Geometry check sheet. Reference: the model listing, model coordinates, mm. A direction names the side the tool comes from. Round coordinates to 2 decimals unless told otherwise and drop trailing zeros. Write each loop counter-clockwise with the first axis right and the second up, starting at its lowest first coordinate (ties: lowest second). Pieces come first, ordered by that corner, then holes. Notation, with made-up numbers: (81.25, 51) -> (132.25, 51) arc R32 ccw to (132.25, 81) -> close; hole circle Ø1 at (23.25, -12). An arc over 180 degrees is marked (long way). Use a Markdown table: item, result.
```python
from build123d import *

# Parameters (mm, degrees)
CROQUIS1_W              = 29
CROQUIS1_H              = 46
SALIENTE_EXTRUIR1_DEPTH = 4
CROQUIS2_W              = 5
CROQUIS2_H              = 29
SALIENTE_EXTRUIR2_DEPTH = 7
CROQUIS3_W              = 5
CROQUIS3_H              = 29
SALIENTE_EXTRUIR3_DEPTH = 21
CROQUIS4_W              = 29
CROQUIS4_H              = 15
SALIENTE_EXTRUIR4_DEPTH = 28
CROQUIS5_R              = 1.5
CORTAR_EXTRUIR1_DEPTH   = 28
CROQUIS6_W              = 28
CROQUIS6_H              = 10
CORTAR_EXTRUIR2_DEPTH   = 60
CORTAR_EXTRUIR3_START   = -5
CROQUIS7_W              = 4.510634874
CROQUIS7_H              = 12.04330307
CORTAR_EXTRUIR3_DEPTH   = 60
CORTAR_EXTRUIR4_START   = -5
CROQUIS8_W              = 3.464680309
CROQUIS8_H              = 12
CORTAR_EXTRUIR4_DEPTH   = 60


with BuildPart() as part:
    # Croquis1 → Saliente-Extruir1 (new body)
    with BuildSketch(Plane(origin=(0, 0, 0), x_dir=(0, 1, 0), z_dir=(0, 0, 1))):
        Rectangle(CROQUIS1_W, CROQUIS1_H)
    extrude(amount=SALIENTE_EXTRUIR1_DEPTH)



with BuildPart() as body_2:
    # Croquis2 → Saliente-Extruir2 (new body)
    with BuildSketch(Plane.XY.offset(4)):
        with Locations((-25.5, 0)):
            Rectangle(CROQUIS2_W, CROQUIS2_H)
    extrude(amount=SALIENTE_EXTRUIR2_DEPTH)


with BuildPart() as part_1:
    add(part.part)

    add(body_2.part)  # Saliente-Extruir3 merges body 2
    # Croquis3 → Saliente-Extruir3 (add)
    with BuildSketch(Plane(origin=(0, 0, 4), x_dir=(1, 0, 0), z_dir=(0, 0, -1))):
        with Locations((-25.5, 0)):
            Rectangle(CROQUIS3_W, CROQUIS3_H)
    extrude(amount=SALIENTE_EXTRUIR3_DEPTH)

    # Croquis4 → Saliente-Extruir4 (add)
    with BuildSketch(Plane(origin=(-28, 0, 0), x_dir=(0, -1, 0), z_dir=(-1, 0, 0))):
        with Locations((0, -9.5)):
            Rectangle(CROQUIS4_W, CROQUIS4_H)
    extrude(amount=-SALIENTE_EXTRUIR4_DEPTH)

    # Croquis5 → Cortar-Extruir1 (cut)
    with BuildSketch(Plane.XY.offset(4)):
        with Locations((17.5, -9)):
            Circle(CROQUIS5_R)
        with Locations((17.5, 9)):
            Circle(CROQUIS5_R)
        Polygon((-18.5, 0), (-18.5, -6), (4.3, -6), (4.3, 6), (-18.5, 6), align=None)
    extrude(amount=-CORTAR_EXTRUIR1_DEPTH, mode=Mode.SUBTRACT)

    # Croquis6 → Cortar-Extruir2 (cut)
    with BuildSketch(Plane(origin=(0, 14.5, 0), x_dir=(1, 0, 0), z_dir=(0, 1, 0))):
        with Locations((-14, 12)):
            Rectangle(CROQUIS6_W, CROQUIS6_H)
    extrude(amount=-CORTAR_EXTRUIR2_DEPTH, mode=Mode.SUBTRACT)

    # Croquis7 → Cortar-Extruir3 (cut)
    with BuildSketch(Plane.XY.offset(4).offset(CORTAR_EXTRUIR3_START)):
        with Locations((-20.769799618, -0.048913864)):
            Rectangle(CROQUIS7_W, CROQUIS7_H)
    extrude(amount=-CORTAR_EXTRUIR3_DEPTH, mode=Mode.SUBTRACT)

    # Croquis8 → Cortar-Extruir4 (cut)
    with BuildSketch(Plane.XY.offset(4).offset(CORTAR_EXTRUIR4_START)):
        with Locations((-18.492763456, 0)):
            Rectangle(CROQUIS8_W, CROQUIS8_H)
    extrude(amount=-CORTAR_EXTRUIR4_DEPTH, mode=Mode.SUBTRACT)


solid = part_1.part
```
(1) Thickness scan on line 1 (Y direction, x = 17.5, z = 1.55); line 2 (Z direction, x = -3, y = -7.5); line 3 (Y direction, x = -7.5, z = -6). Record the ranges inside material, lowest first.
A:
| item | result |
|---|---|
| line 1 | y = -14.5 to -10.5, -7.5 to 7.5, 10.5 to 14.5 |
| line 2 | z = -7 to -2, 0 to 4 |
| line 3 | y = -14.5 to -6, 6 to 14.5 |
(2) Release check for a two-part mould opening along Y. For faces 1 (the face through (-7, 6, 2)), 2 (the face through (-23.025, 0, -4)), 3 (the face through (-9, 14.5, 2)), 4 (the face through (-12, 10, -2)) record: +Y half, -Y half, draft (parallel to the pull), parting line (faces both ways), or undercut.
A:
| item | result |
|---|---|
| face 1 | undercut |
| face 2 | undercut |
| face 3 | +Y half |
| face 4 | draft |
(3) Gauge pin test, flat ends, axial feed: pin 1 Ø9.5 at (x, y) = (-7, 9) entering from +Z; pin 2 Ø5 at (x, y) = (17.5, -9) entering from -Z; pin 3 Ø5 at (y, z) = (2, -3) entering from +X. Record the tip position at first contact, or that the pin passes through.
A:
| item | result |
|---|---|
| pin 1 | stops at z = 4 |
| pin 2 | stops at z = 0 |
| pin 3 | stops at x = -23 |
(4) Access from +Z, -Z, +X, -X, +Y, -Y to the whole of each face (thin tool, end or side, straight path). Record for faces 5 (the face through (4.3, 0, 2)), 6 (the face through (0, 10, -4)), 7 (the face through (-23, 0, 7)), 8 (the face through (-12, -10, -2)), 9 (the face through (-22, 5.973, -5)).
A:
| item | result |
|---|---|
| face 5 | +Z, -Z |
| face 6 | -Z, +X, +Y, -Y |
| face 7 | +Z, +X, +Y, -Y |
| face 8 | +X, +Y, -Y |
| face 9 | -Z, +X |
(5) Section check D-D on x = 2. Record the cut outline in (y, z), plus the area to 3 significant figures.
A:
| item | result |
|---|---|
| outline | (-14.5, 0) -> (-6, 0) -> (-6, 4) -> (-14.5, 4) -> close; (6, 0) -> (14.5, 0) -> (14.5, 4) -> (6, 4) -> close |
| area | 68.0 mm2 |
(6) Section check B-B on x = -8.5. Record the cut outline in (y, z), plus the area to 3 significant figures.
A:
| item | result |
|---|---|
| outline | (-14.5, -7) -> (-6, -7) -> (-6, -2) -> (-14.5, -2) -> close; (-14.5, 0) -> (-6, 0) -> (-6, 4) -> (-14.5, 4) -> close; (6, -7) -> (14.5, -7) -> (14.5, -2) -> (6, -2) -> close; (6, 0) -> (14.5, 0) -> (14.5, 4) -> (6, 4) -> close |
| area | 153 mm2 |
